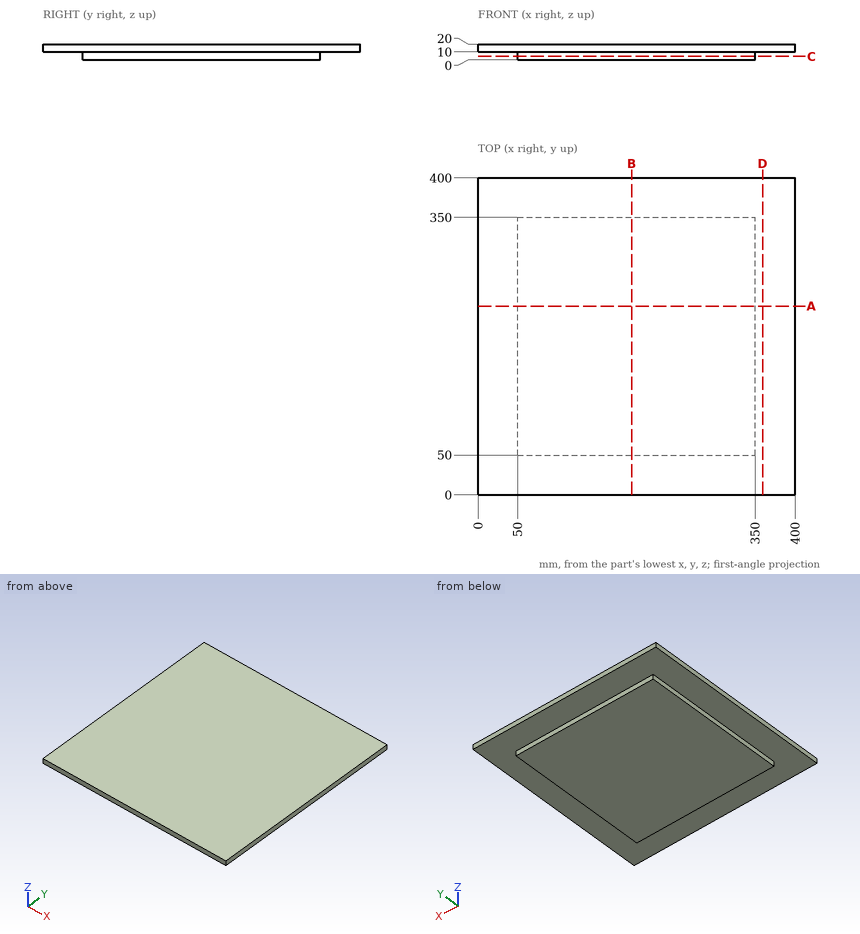
For this review, use the dimensioned drawing (mm, ordinates from the lowest corner) and the shaded views. Coordinates: 2 decimals unless noted, no trailing zeros. Loops run counter-clockwise (first coordinate to the right, second up) from the corner with the lowest first, then second, coordinate; pieces in that order, holes last. Notation, with made-up numbers: (6.25, -11) -> (32.25, -11) arc R21 cw to (32.25, 11) -> close; hole circle Ø8 at (-21.75, -33.5). An arc over 180 degrees is marked (long way). Use a Markdown table: item, result. Add a question column.
1. To check wall thickness, follow line 1 (X direction, y = 89.5, z = 1.5); line 2 (Z direction, x = 71, y = 353.5). State the ranges of each line that lie inside material, in increasing order.
2. Add section C-C on z = 4.5. Write out the cut boundary in (x, y).
3. Clearance check with flat-ended pins moving along their axes: pin 1 Ø1 at (y, z) = (185.5, 3) entering from -X; pin 2 Ø2 at (y, z) = (78.5, 8.5) entering from +X; pin 3 Ø2 at (x, z) = (66, 3.5) entering from -Y. State where each tip first meets the part, or that it passes through.
4. Add section A-A on y = 238. Write out the cut boundary in (x, z), plus the area to 3 significant figures.
5. Add section D-D on x = 359. Write out the cut boundary in (y, z).
Returned:
| question | item | result |
|---|---|---|
| 1 | line 1 | x = 50 to 350 |
| 1 | line 2 | z = 10 to 20 |
| 2 | outline | (50, 50) -> (350, 50) -> (350, 350) -> (50, 350) -> close |
| 3 | pin 1 | stops at x = 50 |
| 3 | pin 2 | stops at x = 350 |
| 3 | pin 3 | stops at y = 50 |
| 4 | outline | (0, 10) -> (50, 10) -> (50, 0) -> (350, 0) -> (350, 10) -> (400, 10) -> (400, 20) -> (0, 20) -> close |
| 4 | area | 7,000 mm² |
| 5 | outline | (0, 10) -> (400, 10) -> (400, 20) -> (0, 20) -> close |
